```python
from build123d import *

# Parameters (mm, degrees)
ESQUISSE2_R                   = 50
BOSS_EXTRU_1_DEPTH            = 200
ENL_V_MAT_EXTRU_1_DEPTH       = 213.132034356
ENL_V_MAT_EXTRU_1_DEPTH_BACK  = 213.132034356
ESQUISSE3_R                   = 6.25
ENL_V_START                   = -100
ESQUISSE4_R                   = 45
ENL_V_MAT_EXTRU_2_DEPTH       = 507.201920355
ENL_V_MAT_EXTRU_11_DEPTH      = 230.128784901
ENL_V_MAT_EXTRU_11_DEPTH_BACK = 49


with BuildPart() as part:
    # Esquisse2 → Boss.-Extru.1 (new, symmetric)
    with BuildSketch(Plane.XY):
        Circle(ESQUISSE2_R)
    extrude(amount=BOSS_EXTRU_1_DEPTH, both=True)

    # Esquisse3 → Enlèv. mat.-Extru.1 (cut, two sides: drawn at the far end of the back side and taken through both)
    with BuildSketch(Plane(origin=(0, 0, 0), x_dir=(0, 0, -1), z_dir=(1, 0, 0)).offset(-ENL_V_MAT_EXTRU_1_DEPTH_BACK)):
        Circle(ESQUISSE3_R)
    extrude(amount=ENL_V_MAT_EXTRU_1_DEPTH + ENL_V_MAT_EXTRU_1_DEPTH_BACK, mode=Mode.SUBTRACT)

    # Esquisse4 → Enlèv. mat.-Extru.2 (cut)
    with BuildSketch(Plane.XY.offset(200).offset(ENL_V_START)):
        with Locations(Location((0, 0, 0), (0, 0, 180))):
            Circle(ESQUISSE4_R)
    enl_v_mat_extru_2 = extrude(amount=ENL_V_MAT_EXTRU_2_DEPTH, mode=Mode.SUBTRACT)

    # Symétrie1: Enlèv. mat.-Extru.2 across plane
    add(enl_v_mat_extru_2.mirror(Plane.XY), mode=Mode.SUBTRACT)

    # Esquisse5 → Enlèv. mat.-Extru.11 (cut, two sides: drawn at the far end of the back side and taken through both)
    with BuildSketch(Plane(origin=(50, 0, 0), x_dir=(0, 0, -1), z_dir=(1, 0, 0)).offset(-ENL_V_MAT_EXTRU_11_DEPTH_BACK)):
        with BuildLine():
            Line((-156.140277695, -10), (-156.140277695, -40))
            ThreePointArc((-156.140277695, -40), (-166.140277695, -50), (-176.140277695, -40))
            Line((-176.140277695, -40), (-176.140277695, -10))
            ThreePointArc((-176.140277695, -10), (-166.140277695, 0), (-156.140277695, -10))
        make_face()
    extrude(amount=ENL_V_MAT_EXTRU_11_DEPTH + ENL_V_MAT_EXTRU_11_DEPTH_BACK, mode=Mode.SUBTRACT)


solid = part.part
```
Input: part model. Units: mm. Frame: model coordinates. A direction names the side the tool comes from. Round coordinates to 2 decimals unless told otherwise and drop trailing zeros. Loops run counter-clockwise (first coordinate to the right, second up) from the corner with the lowest first, then second, coordinate; pieces in that order, holes last. Notation, with made-up numbers: M 35.25,-33.75 L 86.25,-33.75 A27 cw 86.25,-7.75 Z; hole C 8,-6 d6. An arc over 180 degrees is marked long. Answer in a Markdown table with one row per item. Add a question column.
1. Set-up query: faces 1 (the face through (-0.7, 1.88, -5.96)), 2 (the face through (1, -1, 100)), 3 (the face through (38, -26, 176.14)), 4 (the face through (48, 0, 166)), 5 (the face through (-20.765, 39.923, -149.3)). Return all of +Z, -Z, +X, -X, +Y, -Y with unobstructed straight access to the full face (end or side cutting, diameter ignored); none if empty.
2. Mould query, pull axis X, two halves, no side actions, for faces 6 (the face through (-41, 19, 200)), 7 (the face through (47.69, 15.02, 2.8)), 8 (the face through (1, -1, -100)), 9 (the face through (-20.765, 39.923, 149.3)). Classes: released by +X, released by -X, zero draft, split by the parting line, or undercut.
3. Section B-B (x = -7). Output: boundary loops of the cut face in (y, z).
4. Section A-A (x = 8). Output: boundary loops of the cut face in (y, z).
5. Section C-C (z = -171.5). Output: boundary loops of the cut face in (x, y), and give its area (3 significant figures).
6. Section D-D (y = 20). Output: boundary loops of the cut face in (x, z).
7. Contact query for flat-ended pins moving along their axis: pin 1 (4 mm diameter, centred on y = 27.5, z = 35.5, fed in from -X); pin 2 (6 mm diameter, centred on y = -6, z = 64, fed in from +X); pin 3 (2.5 mm diameter, centred on y = -47.5, z = 169, fed in from +X); pin 4 (11 mm diameter, centred on y = 0, z = 0, fed in from -X). Output: stop coordinate, or through.
8. Ray query, probe 1 along Y at (x, z) = (0, 131); probe 2 along Z at (x, y) = (-24.5, 0). Return the intervals inside material, ascending.
Values follow:
| question | item | result |
|---|---|---|
| 1 | face 1 | +X, -X |
| 1 | face 2 | +Z |
| 1 | face 3 | +X |
| 1 | face 4 | +X, -Y |
| 1 | face 5 | -Z |
| 2 | face 6 | zero draft |
| 2 | face 7 | split by the parting line |
| 2 | face 8 | undercut |
| 2 | face 9 | undercut |
| 3 | outline | M -49.51,-200 L -44.45,-200 L -44.45,-100 L 44.45,-100 L 44.45,-200 L 49.51,-200 L 49.51,200 L 44.45,200 L 44.45,100 L -44.45,100 L -44.45,200 L -49.51,200 Z; hole C 0,0 d12.5 |
| 4 | outline | M -49.36,-200 L -44.28,-200 L -44.28,-100 L 44.28,-100 L 44.28,-200 L 49.36,-200 L 49.36,200 L 44.28,200 L 44.28,100 L -44.28,100 L -44.28,157.1 A10 cw -49.36,162.61 Z; M -49.36,169.67 A10 cw -44.28,175.18 L -44.28,200 L -49.36,200 Z; hole C 0,0 d12.5 |
| 5 | outline | C 0,0 d100; hole C 0,0 d90 |
| 5 | area | 1,490 mm^2 |
| 6 | outline | M -45.83,-200 L -40.31,-200 L -40.31,-100 L 40.31,-100 L 40.31,-200 L 45.83,-200 L 45.83,200 L 40.31,200 L 40.31,100 L -40.31,100 L -40.31,200 L -45.83,200 Z |
| 7 | pin 1 | x = -43.01 |
| 7 | pin 2 | x = 49.91 |
| 7 | pin 3 | x = 1 |
| 7 | pin 4 | through |
| 8 | probe 1 | -50 to -45, 45 to 50 |
| 8 | probe 2 | -100 to -6.25, 6.25 to 100 |
